```python
from build123d import *

# Parameters (mm, degrees)
F0_W     = 30
F0_H     = 50
F1_DEPTH = 30


with BuildPart() as f1:
    # F0 (on Top) → F1 (new body)
    with BuildSketch(Plane.XY):
        Rectangle(F0_W, F0_H)
    extrude(amount=F1_DEPTH)

    # F4: sweep along a path in F3
    with BuildLine(Plane.YZ.offset(15)) as f4_path:
        Line((25, 30), (-25, 10))
    # F2 (on face) → F4 (sweep, cut)
    with BuildSketch(Plane.XZ.offset(25)):
        Polygon((15, 30), (-5, 30), (15, 10), align=None)
        Polygon((-15, 30), (-15, 10), (-5, 30), align=None)
    sweep(path=f4_path.line, mode=Mode.SUBTRACT)


solid = f1.part
```
For this review, take the finished solid that the model builds, in its own axes (mm). Give positions to 0.01 mm unless a question says otherwise; leave off trailing zeros. Write each loop counter-clockwise with the first axis right and the second up, starting at its lowest first coordinate (ties: lowest second). Pieces come first, ordered by that corner, then holes.
Item 1: Take a section at C-C (y = -5.5). Give the boundary of the cut face in (x, z).
Item 2: Take a section at D-D (x = -8). Give the boundary of the cut face in (y, z), and give its area (4 significant figures).
Item 3: Wall thickness on probe 1 along X at (y, z) = (5, 22.5); probe 2 along Z at (x, y) = (9.5, -14); probe 3 along Z at (x, y) = (10, 12): over which ranges is each line inside the solid? List them lowest first.
Item 4: Take a section at B-B (z = 24). Give the boundary of the cut face in (x, y).
Item 5: Take a section at A-A (x = -11.5). Give the boundary of the cut face in (y, z).
Established:
1. outline: (-15, 0) - (15, 0) - (15, 17.8) - (2.8, 30) - (-8.9, 30) - (-15, 17.8) - close
2. outline: (-25, 0) - (25, 0) - (25, 30) - (-10, 30) - (-25, 24) - close
2. area: 1,455 mm2
3. probe 1: x = -14.75 to 14.5
3. probe 2: z = 0 to 19.9
3. probe 3: z = 0 to 29.8
4. outline: (-15, 10) - (-8, -25) - (1, -25) - (15, 10) - (15, 25) - (-15, 25) - close
5. outline: (-25, 0) - (25, 0) - (25, 30) - (7.5, 30) - (-25, 17) - close
